Here's how the part is built. I have some questions about the finished solid (model axes, mm). Coordinates: 2 decimals unless noted, no trailing zeros. Loops run counter-clockwise (first coordinate to the right, second up) from the corner with the lowest first, then second, coordinate; pieces in that order, holes last. Notation, with made-up numbers: M 19.5,61 L 45.5,61 A7 ccw 45.5,71 Z; hole C -15.75,-24 d7. An arc over 180 degrees is marked long. Use CSV: the item, a comma, the result in double quotes. Start each with the question number.
Q1. For pin 1 Ø1 at (x, y) = (7.5, -5.5) entering from +Z; pin 2 Ø3 at (x, y) = (5, 3) entering from -Z; pin 3 Ø1 at (y, z) = (4, 3) entering from -X; pin 4 Ø4 at (x, y) = (4, -5.5) entering from +Z, each with a flat end and sliding along its axis, tell me the tip position at first contact or that it passes through.
Q2. If we section it at D-D (x = 6.5): Please give me the cut outline in (y, z), and give its area (3 significant figures).
Q3. Please list where these lines run through material, in increasing order: probe 1 along Z at (x, y) = (3.75, 0); probe 2 along Z at (x, y) = (6.5, -2.25); probe 3 along Y at (x, z) = (0.5, 5.5). Write a range as [from, to].
Q4. If we mould it in two halves opening along Y, with no side actions, what happens to faces 1 (the cylindrical face through (0.93, -1.93, -8.68)), 2 (the flat face through (0, 2, -2)), 3 (the cylindrical face through (4.507, 2.435, 0.767))? For each: +Y half, -Y half, draft (parallel to the pull), parting line (faces both ways), or undercut.
Q5. If we section it at C-C (x = 1): Please give me the cut outline in (y, z).
Q6. If we section it at A-A (y = 0): Please give me the cut outline in (x, z) (1 decimal), and give its area (3 significant figures).
from build123d import *


with BuildPart() as part:
    # Sketch1 → Revolve1 (revolve)
    with BuildSketch(Plane.XY):
        with BuildLine():
            Line((0, 2.5527), (8.89, 2.5527))
            Line((8.89, 2.5527), (8.89, 8.89))
            Line((8.89, 8.89), (7.011321947, 8.89))
            Line((7.011321947, 8.89), (6.094778394, 7.3025))
            ThreePointArc((6.094778394, 7.3025), (4.445, 6.35), (2.795221606, 7.3025))
            Line((2.795221606, 7.3025), (1.878678053, 8.89))
            Line((1.878678053, 8.89), (0, 8.89))
            Line((0, 8.89), (0, 2.5527))
        make_face()
    revolve(axis=Axis((0, 0, 0), (1, 0, 0)))


solid = part.part
Results below:
1,pin 1,"z = 7.35"
1,pin 2,"z = -7.48"
1,pin 3,"x = 0"
1,pin 4,"z = 6.97"
2,outline,"C 0,0 d16.01; hole C 0,0 d5.11"
2,area,"181 mm^2"
3,probe 1,"[-6.48, -2.55], [2.55, 6.48]"
3,probe 2,"[-7.68, -1.21], [1.21, 7.68]"
3,probe 3,"[-6.98, 6.98]"
4,face 1,"parting line"
4,face 2,"draft"
4,face 3,"undercut"
5,outline,"C 0,0 d17.78; hole C 0,0 d5.11"
6,outline,"M 0,-8.9 L 1.9,-8.9 L 2.8,-7.3 A1.9 cw 6.1,-7.3 L 7,-8.9 L 8.9,-8.9 L 8.9,-2.6 L 0,-2.6 Z; M 0,2.6 L 8.9,2.6 L 8.9,8.9 L 7,8.9 L 6.1,7.3 A1.9 cw 2.8,7.3 L 1.9,8.9 L 0,8.9 Z"
6,area,"94.8 mm^2"
